Part model, mm, in its own coordinate system. Face numbers are marked on the shaded views. A direction names the side the tool comes from. Coordinates: 2 decimals unless noted, no trailing zeros. Write each loop counter-clockwise with the first axis right and the second up, starting at its lowest first coordinate (ties: lowest second). Pieces come first, ordered by that corner, then holes. Notation, with made-up numbers: (11.5, 86) -> (61.5, 86) arc R19 ccw to (61.5, 90) -> close; hole circle Ø7 at (69, -38.5). An arc over 180 degrees is marked (long way). Write item = value, one per line. Start each with the question number.
Q1. Band-saw the part on A-A, the plane x = 30. List the corners of the cut face in (y, z).
Q2. Pin check, flat tips, straight feed: P1, Ø0.9, axis at y = 15, z = 1, coming from the +X side; P2, Ø9, axis at y = 14.5, z = 19.5, coming from the -X side; P3, Ø3, axis at x = 30, y = 5, coming from the +Z side; P4, Ø10, axis at y = 15.5, z = 18, coming from the +X side. Stop position of each tip, or through.
Q3. Tool access for the marked faces 4, 5, 6, 7 and 8: list every direction of +Z, -Z, +X, -X, +Y, -Y with a clear straight run to the whole face (end or side of a thin tool).
Q4. Band-saw the part on B-B, the plane y = 14.5. List the corners of the cut face in (x, z), plus the area to 4 significant figures.
Q5. Pull direction Z, two halves, no side cores. Call the marked faces 1, 2 and 3: released by +Z, released by -Z, zero draft, split by the parting line, or undercut.
Q6. Probe line 1 (X direction, y = 13, z = 7.5); line 2 (Z direction, x = 13.6, y = 14.5); line 3 (Y direction, x = 10, z = 1.9). List the from-to ranges inside material, lowest first.
Q7. Band-saw the part on C-C, the plane x = 38.5. List the corners of the cut face in (y, z).
Q8. Band-saw the part on D-D, the plane y = 5. List the corners of the cut face in (x, z).
from build123d import *

# Parameters (mm, degrees)
SKETCH1_W               = 7
SKETCH1_H               = 9
BOSS_EXTRUDE2_DEPTH     = 32
SKETCH1_4_R             = 2.5
BOSS_EXTRUDE3_DEPTH     = 3
CUT_EXTRUDE1_DEPTH      = 55.635153519
CUT_EXTRUDE1_DEPTH_BACK = 55.635153519
SKETCH3_W               = 11
SKETCH3_H               = 27.5
SKETCH6_W               = 23
SKETCH6_H               = 9
BOSS_EXTRUDE4_DEPTH     = 19
CUT_EXTRUDE3_DEPTH      = 60.16924877
CUT_EXTRUDE3_DEPTH_BACK = 60.16924877
SKETCH9_W               = 19
SKETCH9_H               = 20
CUT_EXTRUDE4_DEPTH      = 51.129831438
CUT_EXTRUDE4_DEPTH_BACK = 51.129831438
SKETCH12_R              = 4
SKETCH14_W              = 13
SKETCH14_H              = 10
BOSS_EXTRUDE6_DEPTH     = 60
SKETCH17_W              = 11.5
SKETCH17_H              = 8.5
CUT_EXTRUDE6_DEPTH      = 58.5
SKETCH18_W              = 13
SKETCH18_H              = 1.5
BOSS_EXTRUDE7_DEPTH     = 8
SKETCH19_R              = 3
CUT_EXTRUDE7_DEPTH      = 1.5
SKETCH20_W              = 8.5
SKETCH20_H              = 35
CUT_EXTRUDE8_DEPTH      = 1.5
FILLET1_R               = 10


with BuildPart() as part:
    # Sketch1 → Boss-Extrude2 (new body)
    with BuildSketch(Plane.XY):
        with Locations((23.5, 14.5)):
            Rectangle(SKETCH1_W, SKETCH1_H)
        with Locations((16.5, 14.5)):
            Rectangle(SKETCH1_W, SKETCH1_H)
    extrude(amount=BOSS_EXTRUDE2_DEPTH)

    # Sketch1<4> → Boss-Extrude3 (add)
    # profile 1 of 2: a face of its own
    with BuildSketch(Plane.XY):
        Polygon((0, 0), (20, 0), (20, 10), (13, 10), (13, 19), (20, 19), (20, 20), (0, 20), align=None)
        with Locations((10, 5)):
            Circle(SKETCH1_4_R, mode=Mode.SUBTRACT)
    # profile 2 of 2: a face of its own
    with BuildSketch(Plane.XY):
        Polygon((20, 10), (20, 0), (40, 0), (40, 20), (20, 20), (20, 19), (27, 19), (27, 10), align=None)
        with Locations((30, 5)):
            Circle(SKETCH1_4_R, mode=Mode.SUBTRACT)
    extrude(amount=BOSS_EXTRUDE3_DEPTH)

    # Sketch3 → Cut-Extrude1 (cut, two sides: drawn at the far end of the back side and taken through both)
    with BuildSketch(Plane(origin=(0, 19, 0), x_dir=(1, 0, 0), z_dir=(0, 1, 0)).offset(-CUT_EXTRUDE1_DEPTH_BACK)):
        with Locations((20, -16.75)):
            Rectangle(SKETCH3_W, SKETCH3_H)
    extrude(amount=CUT_EXTRUDE1_DEPTH + CUT_EXTRUDE1_DEPTH_BACK, mode=Mode.SUBTRACT)

    # Sketch6 → Boss-Extrude4 (add)
    with BuildSketch(Plane(origin=(27, 0, 0), x_dir=(0, 0, -1), z_dir=(1, 0, 0))):
        with Locations((-20.5, 14.5)):
            Rectangle(SKETCH6_W, SKETCH6_H)
    extrude(amount=BOSS_EXTRUDE4_DEPTH)

    # Sketch9 → Cut-Extrude3 (cut, two sides: drawn at the far end of the back side and taken through both)
    with BuildSketch(Plane(origin=(0, 19, 0), x_dir=(1, 0, 0), z_dir=(0, 1, 0)).offset(-CUT_EXTRUDE3_DEPTH_BACK)):
        with Locations((35, -20.5)):
            Rectangle(SKETCH9_W, SKETCH9_H)
    extrude(amount=CUT_EXTRUDE3_DEPTH + CUT_EXTRUDE3_DEPTH_BACK, mode=Mode.SUBTRACT)

    # Sketch12 → Cut-Extrude4 (cut, two sides: drawn at the far end of the back side and taken through both)
    with BuildSketch(Plane.ZY.offset(-13).offset(-CUT_EXTRUDE4_DEPTH_BACK)):
        with Locations(Location((19.5, 14.5, 0), (0, 0, 270))):
            Circle(SKETCH12_R)
    extrude(amount=CUT_EXTRUDE4_DEPTH + CUT_EXTRUDE4_DEPTH_BACK, mode=Mode.SUBTRACT)

    # Sketch14 → Boss-Extrude6 (add)
    with BuildSketch(Plane(origin=(0, 19, 0), x_dir=(1, 0, 0), z_dir=(0, 1, 0))):
        with Locations((19.5, -27)):
            Rectangle(SKETCH14_W, SKETCH14_H)
    extrude(amount=BOSS_EXTRUDE6_DEPTH)

    # Sketch17 → Cut-Extrude6 (cut)
    with BuildSketch(Plane.XZ.offset(-19)):
        with Locations((20.25, 26.25)):
            Rectangle(SKETCH17_W, SKETCH17_H)
    extrude(amount=-CUT_EXTRUDE6_DEPTH, mode=Mode.SUBTRACT)

    # Sketch18 → Boss-Extrude7 (add)
    with BuildSketch(Plane(origin=(0, 0, 22), x_dir=(-1, 0, 0), z_dir=(0, 0, -1))):
        with Locations((-19.5, 78.25)):
            Rectangle(SKETCH18_W, SKETCH18_H)
    extrude(amount=BOSS_EXTRUDE7_DEPTH)

    # Sketch19 → Cut-Extrude7 (cut)
    with BuildSketch(Plane(origin=(0, 79, 0), x_dir=(1, 0, 0), z_dir=(0, 1, 0))):
        with Locations(Location((20.2198624, -20.303001359, 0), (0, 0, 270))):
            Circle(SKETCH19_R)
    extrude(amount=-CUT_EXTRUDE7_DEPTH, mode=Mode.SUBTRACT)

    # Sketch20 → Cut-Extrude8 (cut)
    with BuildSketch(Plane(origin=(14.5, 0, 0), x_dir=(0, 0, -1), z_dir=(1, 0, 0))):
        with Locations((-26.25, 60)):
            Rectangle(SKETCH20_W, SKETCH20_H)
    extrude(amount=-CUT_EXTRUDE8_DEPTH, mode=Mode.SUBTRACT)

    # Fillet1
    # the kernel refuses this fillet: 10 mm, written as the material it adds along each edge
    with BuildSketch(Plane(origin=(14.5, 42.5, 30.5), x_dir=(0, 0, -1), z_dir=(-1, 0, 0))) as fillet1_piece_1:
        with BuildLine():
            CenterArc((10, -9.886859967), FILLET1_R, 98.626926559, 81.373073441)
            Line((0, -9.886859967), (-0.2, -9.886859967))
            Line((-0.2, -9.886859967), (-0.2, 0))
            Line((-0.2, 0), (0, 0.2))
            ThreePointArc((0, 0.2), (4.25, 0.2), (8.47, 0.197737199))
            Line((8.47, 0.197737199), (8.5, 0))
        make_face()
    extrude(amount=1.5)


solid = part.part
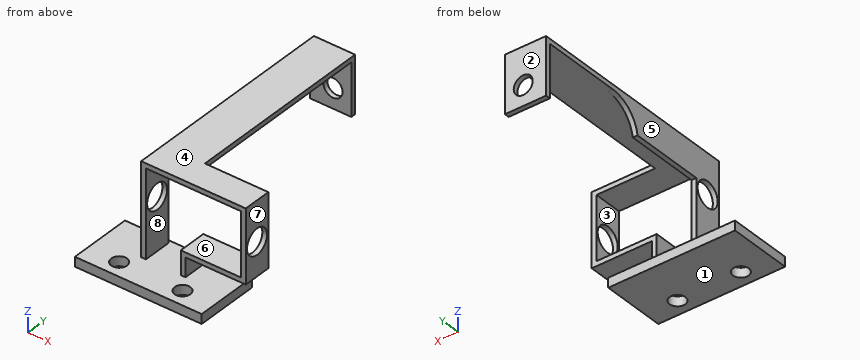
Ans:
q1.outline = (0, 0) -> (2.5, 0) -> (2.5, 3) -> (0, 3) -> close; (7.5, 0) -> (20, 0) -> (20, 3) -> (7.5, 3) -> close; (10, 9) -> (19, 9) -> (19, 10.5) -> (10, 10.5) -> close; (10, 30.5) -> (19, 30.5) -> (19, 32) -> (10, 32) -> close
q2.P1 = 40
q2.P2 = 13
q2.P3 = through
q2.P4 = 46
q3.face_4 = +Z, +X, -X, +Y, -Y
q3.face_5 = +Z, -X, +Y, -Y
q3.face_6 = +Y, -Y
q3.face_7 = +Z, -Z, +X, +Y, -Y
q3.face_8 = -Y
q4.outline = (0, 0) -> (40, 0) -> (40, 3) -> (27, 3) -> (27, 9) -> (46, 9) -> (46, 15.5) -> (44.5, 15.5) -> (44.5, 10.5) -> (25.5, 10.5) -> (25.5, 3) -> (14.5, 3) -> (14.5, 15.5) -> (13, 15.5) -> (13, 3) -> (0, 3) -> close; (13, 23.5) -> (14.5, 23.5) -> (14.5, 30.5) -> (44.5, 30.5) -> (44.5, 23.5) -> (46, 23.5) -> (46, 32) -> (13, 32) -> close
q4.area = 256.5 mm2
q5.face_1 = released by -Z
q5.face_2 = zero draft
q5.face_3 = undercut
q6.line_1 = 13 to 14.5, 25.5 to 27
q6.line_2 = 0 to 15.5, 23.5 to 32
q6.line_3 = 0 to 2.5, 7.5 to 20
q7.outline = (0, 0) -> (20, 0) -> (20, 3) -> (0, 3) -> close; (10, 9) -> (19, 9) -> (19, 10.5) -> (10, 10.5) -> close; (10, 30.5) -> (19, 30.5) -> (19, 32) -> (10, 32) -> close
q8.outline = (0, 0) -> (7.5, 0) -> (7.5, 3) -> (0, 3) -> close; (12.5, 0) -> (27.5, 0) -> (27.5, 3) -> (12.5, 3) -> close; (32.5, 0) -> (40, 0) -> (40, 3) -> (32.5, 3) -> close
